```python
from build123d import *

# Parameters (mm, degrees)
F0_R     = 15.5
F1_DEPTH = 30
F2_W     = 51
F2_H     = 51
F3_DEPTH = 1
F4_W     = 51
F4_H     = 51
F4_W_2   = 31
F4_H_2   = 31
F5_DEPTH = 30.5


with BuildPart() as f1:
    # F0 (on Top) → F1 (new body)
    with BuildSketch(Plane.XY):
        Circle(F0_R)
    extrude(amount=F1_DEPTH)

    # F2 (on face) → F3 (join)
    with BuildSketch(Plane(origin=(0, 0, 0), x_dir=(1, 0, 0), z_dir=(0, 0, -1))):
        Rectangle(F2_W, F2_H)
        Polygon((15.5, 0), (15.5, -15.5), (0, -15.5), (-15.5, -15.5), (-15.5, 0), (-15.5, 15.5), (-6.64e-08, 15.5), (15.5, 15.5), align=None, mode=Mode.SUBTRACT)
        with BuildLine():
            Line((0, -15.5), (15.5, -15.5))
            Line((15.5, -15.5), (15.5, 0))
            ThreePointArc((15.5, 0), (10.9601551084, -10.9601551084), (0, -15.5))
        make_face()
        with BuildLine():
            Line((-15.5, -15.5), (0, -15.5))
            ThreePointArc((0, -15.5), (-10.9601551084, -10.9601551084), (-15.5, 0))
            Line((-15.5, 0), (-15.5, -15.5))
        make_face()
        with BuildLine():
            ThreePointArc((-15.5, 0), (-10.9601551084, -10.9601551084), (0, -15.5))
            ThreePointArc((0, -15.5), (10.9601551084, -10.9601551084), (15.5, 0))
            ThreePointArc((15.5, 0), (10.9601550849, 10.9601551319), (-6.64e-08, 15.5))
            ThreePointArc((-6.64e-08, 15.5), (-10.9601551319, 10.9601550849), (-15.5, 0))
        make_face()
        with BuildLine():
            ThreePointArc((-6.64e-08, 15.5), (10.9601550849, 10.9601551319), (15.5, 0))
            Line((15.5, 0), (15.5, 15.5))
            Line((15.5, 15.5), (-6.64e-08, 15.5))
        make_face()
        with BuildLine():
            Line((-15.5, 15.5), (-15.5, 0))
            ThreePointArc((-15.5, 0), (-10.9601551319, 10.9601550849), (-6.64e-08, 15.5))
            Line((-6.64e-08, 15.5), (-15.5, 15.5))
        make_face()
    extrude(amount=F3_DEPTH)

    # F4 (on face) → F5 (join)
    with BuildSketch(Plane(origin=(0, 0, -1), x_dir=(1, 0, 0), z_dir=(0, 0, -1))):
        Rectangle(F4_W, F4_H)
        Rectangle(F4_W_2, F4_H_2, mode=Mode.SUBTRACT)
    extrude(amount=F5_DEPTH)


solid = f1.part
```
Design review of the part built by this model. Coordinates are the model's own, in mm. A direction names the side the tool comes from. Coordinates: 2 decimals unless noted, no trailing zeros. Write each loop counter-clockwise with the first axis right and the second up, starting at its lowest first coordinate (ties: lowest second). Pieces come first, ordered by that corner, then holes.
1) Add section C-C (z = 26.5). Write out the cut boundary in (x, y), plus the area to 3 significant figures.
2) Mouldability with a two-part tool opening along Y and no side actions: class faces 1 (the flat face through (0, 25.5, -16)), 2 (the flat face through (17, 0, -31.5)), 3 (the flat face through (15.5, 0, -16)) as +Y half, -Y half, draft (parallel to the pull), parting line (faces both ways), or undercut.
3) Machinability: for faces 4 (the flat face through (25.5, 0, -16)), 5 (the cylindrical face through (-2.018, 15.368, 14.79)), 6 (the flat face through (0, 15.5, -16)), which of the approach directions +Z, -Z, +X, -X, +Y, -Y give a long, thin tool a straight path to every point of the face, cutting with its end or side? Answer none if there is none.
4) Add section A-A (x = 0). Write out the cut boundary in (y, z).
5) To check wall thickness, follow L1, parallel to Y at x = 4, z = -28; L2, parallel to Z at x = 13, y = 23. State the ranges of each line that lie inside material, in increasing order.
6) Insertion check: pin 1 (9.5 mm diameter, centred on x = -5, y = -4.5, fed in from -Z); pin 2 (2 mm diameter, centred on y = 13.5, z = 4.5, fed in from -X); pin 3 (1 mm diameter, centred on x = 7.5, z = 18.5, fed in from +Y). Each pin has a flat end and moves straight along its axis. Give the tip position at first contact, or say it passes through.
7) Add section D-D (y = 19.5). Write out the cut boundary in (x, z).
Check result:
1. outline: circle Ø31 at (0, 0)
1. area: 755 mm2
2. face 1: +Y half
2. face 2: draft
2. face 3: undercut
3. face 4: +Z, -Z, +X, +Y, -Y
3. face 5: +Z
3. face 6: -Z
4. outline: (-25.5, -31.5) - (-15.5, -31.5) - (-15.5, -1) - (15.5, -1) - (15.5, -31.5) - (25.5, -31.5) - (25.5, 0) - (15.5, 0) - (15.5, 30) - (-15.5, 30) - (-15.5, 0) - (-25.5, 0) - close
5. L1: y = -25.5 to -15.5, 15.5 to 25.5
5. L2: z = -31.5 to 0
6. pin 1: stops at z = -1
6. pin 2: stops at x = -9.17
6. pin 3: stops at y = 13.83
7. outline: (-25.5, -31.5) - (25.5, -31.5) - (25.5, 0) - (-25.5, 0) - close
